```python
from build123d import *

# Parameters (mm, degrees)
CHAMFER1_SIZE = 0.1
FILLET1_R     = 1


with BuildPart() as part:
    # Sketch1 → Revolve1 (revolve)
    with BuildSketch(Plane.XY, mode=Mode.PRIVATE) as revolve1_sk:
        Polygon((4, 0), (4.5, 0), (4.5, 0.5), (6.5, 0.5), (6.5, 0), (7.5, 0), (7.5, 5.15), (7.15, 5.15), (7.15, 6.25), (7.5, 6.25), (7.5, 17.75), (7.15, 17.75), (7.15, 18.85), (7.5, 18.85), (7.5, 24), (6.5, 24), (6.5, 23.5), (4.5, 23.5), (4.5, 24), (4, 24), align=None)
    revolve(revolve1_sk.sketch.rotate(Axis((0, 0, 0), (0, 1, 0)), 90), axis=Axis((0, 0, 0), (0, 1, 0)))

    # Chamfer1
    chamfer1_edges = [part.edges().sort_by_distance(p)[0] for p in [
        (0, 0, 4),
        (0, 0, 4.5),
        (0, 0, 6.5),
        (0, 24, 6.5),
        (0, 24, 4.5),
        (0, 24, 4),
    ]]
    chamfer(chamfer1_edges, length=CHAMFER1_SIZE)

    # Fillet1
    # the kernel refuses this fillet: 1 mm, written as the material it takes off along each edge
    with BuildSketch(Plane(origin=(0, 0, 0), x_dir=(0, 0, -1), z_dir=(1, 0, 0))) as fillet1_piece_1:
        with BuildLine():
            CenterArc((6.5, 0.994987437), FILLET1_R, 275.739170477, 84.260829523)
            Line((7.5, 0.994987437), (7.52, 0.994987437))
            Line((7.52, 0.994987437), (7.52, 0))
            Line((7.52, 0), (7.5, -0.02))
            ThreePointArc((7.5, -0.02), (7.05, -0.02), (6.602, -0.019899749))
            Line((6.602, -0.019899749), (6.6, 0))
        make_face()
    revolve(axis=Axis((0, 0, 0), (0, 1, 0)), mode=Mode.SUBTRACT)
    with BuildSketch(Plane(origin=(0, 24, 0), x_dir=(0, 0, -1), z_dir=(1, 0, 0))) as fillet1_piece_2:
        with BuildLine():
            CenterArc((6.5, -0.994987437), FILLET1_R, 0, 84.260829523)
            Line((7.5, -0.994987437), (7.52, -0.994987437))
            Line((7.52, -0.994987437), (7.52, 0))
            Line((7.52, 0), (7.5, 0.02))
            ThreePointArc((7.5, 0.02), (7.05, 0.02), (6.602, 0.019899749))
            Line((6.602, 0.019899749), (6.6, 0))
        make_face()
    revolve(axis=Axis((0, 24, 0), (0, 1, 0)), mode=Mode.SUBTRACT)


solid = part.part
```
Design review of the part built by this model. Coordinates are the model's own, in mm. A direction names the side the tool comes from. Give positions to 0.01 mm unless a question says otherwise; leave off trailing zeros. Loops run counter-clockwise (first coordinate to the right, second up) from the corner with the lowest first, then second, coordinate; pieces in that order, holes last. Notation, with made-up numbers: M 83,83.25 L 93,83.25 A26 ccw 93,106.25 Z; hole C -28.75,-30 d6. An arc over 180 degrees is marked long. Return JSON: item names as keys, results as strings. Group by question number.
Item 1: Mouldability with a two-part tool opening along Z and no side actions: class faces 4 (the cylindrical face through (-3.04, 0.3, 3.32)), 5 (the cylindrical face through (-7.09, 5.71, 0.93)) as released by +Z, released by -Z, zero draft, split by the parting line, or undercut.
Item 2: For probe 1 along X at (y, z) = (14, 0); probe 2 along X at (y, z) = (0.3, 0); probe 3 along X at (y, z) = (21, -6), list the stretches that pass through material, from the lowest coordinate up.
Item 3: We need section A-A (y = 20). Give the boundary of the cut face in (x, z).
Item 4: Tool access review of faces 1 (the cylindrical face through (3.955, 0.297, 5.158)), 2 (the cylindrical face through (-3.04, 23.7, 3.32)), 3 (the cylindrical face through (-7.09, 18.31, 0.93)): name each direction out of +Z, -Z, +X, -X, +Y, -Y from which nothing blocks a thin tool from reaching the whole face with its end or side.
Item 5: Insertion check: pin 1 Ø6 at (y, z) = (2.5, -2.5) entering from -X; pin 2 Ø3 at (y, z) = (3.5, -3) entering from -X; pin 3 Ø2 at (x, y) = (-5, 3) entering from -Z. Each pin has a flat end and moves straight along its axis. Give the tip position at first contact, or say it passes through.
Output:
{
 "1": {"face 4": "undercut", "face 5": "split by the parting line"},
 "2": {"probe 1": "x = -7.5 to -4, 4 to 7.5", "probe 2": "x = -7.22 to -6.5, -4.5 to -4, 4 to 4.5, 6.5 to 7.22", "probe 3": "x = -4.5 to 4.5"},
 "3": {"outline": "C 0,0 d15; hole C 0,0 d8"},
 "4": {"face 1": "-Y", "face 2": "+Y", "face 3": "none"},
 "5": {"pin 1": "stops at x = -7.5", "pin 2": "stops at x = -7.35", "pin 3": "stops at z = -6.34"}
}
